Here's how the part is built. I have some questions about the finished solid (model axes, mm). A direction names the side the tool comes from. Round coordinates to 2 decimals unless told otherwise and drop trailing zeros. Write item = value, one per line. Start each with the question number.
(1) If we mould it in two halves opening along Y, with no side actions, what happens to faces 1 (the cylindrical face through (126.7, 7.4, 4.4)), 2 (the flat face through (131.6, 20, 4)), 3 (the flat face through (128, 131.6, 4))? For each: released by +Y, released by -Y, zero draft, split by the parting line, or undercut.
(2) Will these pins go through, and if not, where does the flat tip stop? pin 1 Ø3.5 at (x, z) = (73.5, 3.5) entering from -Y; pin 2 Ø1.6 at (y, z) = (74, 4) entering from -X; pin 3 Ø2.5 at (x, z) = (18.3, 4) entering from +Y; pin 4 Ø2 at (y, z) = (20, 4) entering from +X.
(3) I need wall thicknesses on line 1 along Z through (x, y) = (128, 6); line 2 along X through (y, z) = (133.5, 3); line 3 along X through (y, z) = (11.5, 4). Which ranges of each line are inside material? Lowest first, please.
(4) On a 3-axis mill with a long thin cutter (end or side, diameter ignored), from which of +Z, -Z, +X, -X, +Y, -Y can I reach the whole of each face in a straight line? I mean faces 4 (the flat face through (18, 15, 4)), 5 (the cylindrical face through (138.995, 125.076, 3.368)), 6 (the flat face through (15, 127, 4)). Say none if no direction works.
```python
from build123d import *

# Parameters (mm, degrees)
SKETCH_1_W          = 146.6
SKETCH_1_H          = 146.6
EXTRUDE_1_DEPTH     = 8
SKETCH_2_R          = 1.65
CUT_EXTRUDE_1_DEPTH = 208.477998834
SKETCH_3_R          = 1.65
CUT_EXTRUDE_2_DEPTH = 208.477998834
EXTRUDE_2_REACH     = 209.478
SKETCH_4_W          = 116.6
SKETCH_4_H          = 116.6


with BuildPart() as part:
    # Эскиз1 → Бобышка-Вытянуть1 (new body)
    with BuildSketch(Plane.XY):
        with Locations((73.3, 73.3)):
            Rectangle(SKETCH_1_W, SKETCH_1_H)
    extrude(amount=EXTRUDE_1_DEPTH)

    # Эскиз2 → Вырез-Вытянуть1 (cut, through all)
    with BuildSketch(Plane.XZ):
        with Locations(Location((18.3, 4, 0), (0, 0, 270))):
            Circle(SKETCH_2_R)
        with Locations(Location((73.3, 4, 0), (0, 0, 270))):
            Circle(SKETCH_2_R)
        with Locations(Location((128.3, 4, 0), (0, 0, 270))):
            Circle(SKETCH_2_R)
    extrude(amount=-CUT_EXTRUDE_1_DEPTH, mode=Mode.SUBTRACT)

    # Эскиз3 → Вырез-Вытянуть2 (cut, through all)
    with BuildSketch(Plane.ZY):
        with Locations(Location((4, 20, 0), (0, 0, 270))):
            Circle(SKETCH_3_R)
        with Locations(Location((4, 73.3, 0), (0, 0, 270))):
            Circle(SKETCH_3_R)
        with Locations(Location((4, 126.6, 0), (0, 0, 270))):
            Circle(SKETCH_3_R)
    extrude(amount=-CUT_EXTRUDE_2_DEPTH, mode=Mode.SUBTRACT)

    # Бобышка-Вытянуть2: up to this face of the body (flat: up to its plane)
    extrude_2_end = Plane(part.part.faces().sort_by_distance((73.3, 73.3, 0))[0])
    # Эскиз4 → Бобышка-Вытянуть2 (add, up to the picked face)
    with BuildSketch(Plane.XY.offset(8), mode=Mode.PRIVATE) as extrude_2_sk1:
        with Locations((73.3, 73.3)):
            Rectangle(SKETCH_4_W, SKETCH_4_H)
    extrude_2_tool1 = split(extrude(extrude_2_sk1.sketch, amount=-EXTRUDE_2_REACH, mode=Mode.PRIVATE), bisect_by=extrude_2_end, keep=Keep.BOTH, mode=Mode.PRIVATE)
    add(extrude_2_tool1.solids().sort_by(Axis((73.3, 73.3, 8), (0, 0, -1)))[0])


solid = part.part
```
Returned:
q1.face_1 = zero draft
q1.face_2 = undercut
q1.face_3 = released by +Y
q2.pin_1 = 0
q2.pin_2 = 15
q2.pin_3 = 131.6
q2.pin_4 = 131.6
q3.line_1 = 0 to 2.38, 5.62 to 8
q3.line_2 = 0 to 16.99, 19.61 to 71.99, 74.61 to 126.99, 129.61 to 146.6
q3.line_3 = 0 to 16.65, 19.95 to 71.65, 74.95 to 126.65, 129.95 to 146.6
q4.face_4 = -Y
q4.face_5 = +X
q4.face_6 = -X
